CAD build for the part. Positions are in the model's coordinates, mm. Face numbers are marked on the shaded views. A direction names the side the tool comes from. Coordinates: 2 decimals unless noted, no trailing zeros. Loops run counter-clockwise (first coordinate to the right, second up) from the corner with the lowest first, then second, coordinate; pieces in that order, holes last. Notation, with made-up numbers: (8, 35) -> (43, 35) arc R14 ccw to (43, 52) -> close; hole circle Ø4 at (0.25, 72.25). An arc over 180 degrees is marked (long way). Return JSON: item names as keys, results as strings. Group by question number.
(1) Tool access for the marked faces 4 and 5: list every direction of +Z, -Z, +X, -X, +Y, -Y with a clear straight run to the whole face (end or side of a thin tool).
(2) Saw through at A-A on x = 10.5. Write the cut outline in (y, z).
(3) Saw through at D-D on y = -58. Write the cut outline in (x, z), then the cut area to 3 significant figures.
(4) Probe L1, parallel to X at y = -52.5, z = 52; L2, parallel to X at y = 41, z = 4; L3, parallel to Z at x = -36, y = -9.5. List the from-to ranges inside material, lowest first.
(5) Mould opens along Y. For the marked faces 1, 2 and 3 say: pulls with the +Y half, pulls with the -Y half, needs draft (parallel to the pull), parting line crosses it, or undercut.
(6) Flat gauge pins, fed straight in: pin 1 Ø4 at (x, y) = (0, -56) entering from -Z; pin 2 Ø5 at (x, y) = (41.5, 0) entering from +Z; pin 3 Ø6 at (x, y) = (2.5, 15.5) entering from +Z; pin 4 Ø6 at (x, y) = (-31, -28) entering from -Z. Where does each tip first touch, or does it go through?
(7) Saw through at B-B on y = 0. Give the number of separate pieces and of enclosed holes in the cut face, then the cut area to 3 significant figures.
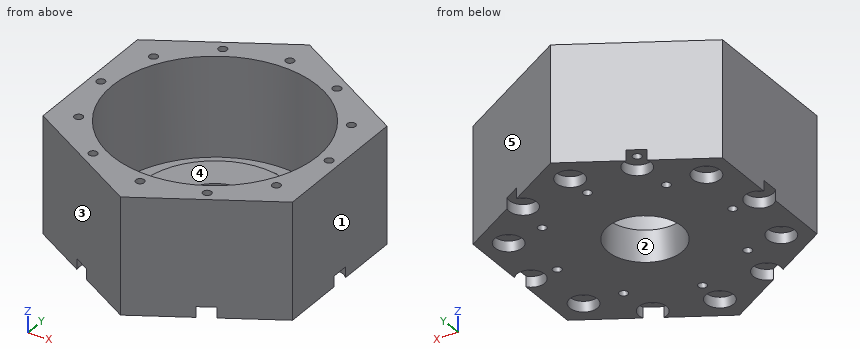
Autodesk Inventor part; units mm, degrees
ref_plane "YZ Plane" through (0, 0, 0) normal (1, 0, 0) x (0, 1, 0)
ref_plane "XZ Plane" through (0, 0, 0) normal (0, 1, 0) x (-1, 0, 0)
ref_plane "XY Plane" through (0, 0, 0) normal (0, 0, 1) x (1, 0, 0)
sketch "Sketch1" plane through (0, 0, 0) normal (0, 0, 1) x (1, 0, 0)
  circle A0 centre (0, 0) radius 17.5
  circle A1 centre (0, 0) radius 67.5
  circle A2 centre (41.5, 0) radius 2
  circle A3 centre (29.3449, 29.3449) radius 2
  circle A4 centre (0, 41.5) radius 2
  circle A5 centre (-29.3449, 29.3449) radius 2
  circle A6 centre (-41.5, 0) radius 2
  circle A7 centre (-29.3449, -29.3449) radius 2
  circle A8 centre (0, -41.5) radius 2
  circle A9 centre (29.3449, -29.3449) radius 2
  dimension "d0" = 35
  dimension "d1" = 135
  dimension "d2" = 4
  dimension "d3" = 41.5
  dimension "d6" = 360
extrude "Extrusion1" add sketch "Sketch1" along normal blind 15
sketch "Sketch5" plane through (0, 0, 15) normal (0, 0, 1) x (1, 0, 0)
  circle A0 centre (0, 0) radius 67.5
  circle A1 centre (0, 0) radius 48.5
  dimension "d19" = 97
extrude "Extrusion4" add sketch "Sketch5" along normal blind 40
sketch "Sketch8" plane through (0, 0, 55) normal (0, 0, 1) x (1, 0, 0)
  circle A0 centre (-54, 0) radius 2
  circle A1 centre (-46.7654, -27) radius 2
  circle A2 centre (-27, -46.7654) radius 2
  circle A3 centre (0, -54) radius 2
  circle A4 centre (27, -46.7654) radius 2
  circle A5 centre (46.7654, -27) radius 2
  circle A6 centre (54, 0) radius 2
  circle A7 centre (46.7654, 27) radius 2
  circle A8 centre (27, 46.7654) radius 2
  circle A9 centre (0, 54) radius 2
  circle A10 centre (-27, 46.7654) radius 2
  circle A11 centre (-46.7654, 27) radius 2
  point P0 (0, 0)
  dimension "d20" = 4
  dimension "d21" = 54
  dimension "d24" = 360
extrude "Extrusion5" cut sketch "Sketch8" against normal through all
sketch "Sketch11" plane through (0, 0, 55) normal (0, 0, 1) x (1, 0, 0)
  line L0 (0, 77.9423) -> (67.5, 38.9711)
  line L1 (67.5, 38.9711) -> (67.5, -38.9711)
  line L2 (67.5, -38.9711) -> (0, -77.9423)
  line L3 (0, -77.9423) -> (-67.5, -38.9711)
  line L4 (-67.5, -38.9711) -> (-67.5, 38.9711)
  line L5 (-67.5, 38.9711) -> (0, 77.9423)
  circle A0 centre (0, 0) radius 67.5
extrude "Extrusion8" add sketch "Sketch11" against normal blind 55 contours L0 A0 L5 | L0 L1 A0 | A0 L4 L5 | L1 L2 A0 | A0 L3 L4 | L2 L3 A0
sketch "Sketch12" plane through (0, 0, 0) normal (0, 0, -1) x (-1, 0, 0)
  circle A0 centre (-54, 0) radius 2
  circle A1 centre (-54, 0) radius 6.5
  circle A2 centre (-46.7654, -27) radius 6.5
  circle A3 centre (-27, -46.7654) radius 6.5
  circle A4 centre (0, -54) radius 6.5
  circle A5 centre (27, -46.7654) radius 6.5
  circle A6 centre (46.7654, -27) radius 6.5
  circle A7 centre (54, 0) radius 6.5
  circle A8 centre (46.7654, 27) radius 6.5
  circle A9 centre (27, 46.7654) radius 6.5
  circle A10 centre (0, 54) radius 6.5
  circle A11 centre (-27, 46.7654) radius 6.5
  circle A12 centre (-46.7654, 27) radius 6.5
  point P0 (0, 0)
  dimension "d37" = 13
  dimension "d40" = 360
extrude "Extrusion9" cut sketch "Sketch12" against normal blind 5 contours A0 | A1 | A2 | A3 | A4 | A5 | A6 | A7 | A8 | A9 | A10 | A11 | A12
sketch "Sketch16" plane through (0, 0, 15) normal (0, 0, 1) x (1, 0, 0)
  circle A0 centre (-41.5, 0) radius 2
  circle A1 centre (0, 0) radius 34.5
  circle A2 centre (0, 0) radius 48.5
  line L0 (-48.5, 0) -> (-34.5, 0)
  circle A3 centre (0, 0) radius 48.5
extrude "Extrusion11" cut sketch "Sketch16" against normal blind 7
sketch "Sketch19" plane through (0, 0, 55) normal (0, 0, 1) x (1, 0, 0)
  circle A0 centre (-27, 46.7654) radius 2
  circle A1 centre (27, 46.7654) radius 2
  circle A2 centre (54, 0) radius 2
  circle A3 centre (27, -46.7654) radius 2
  circle A4 centre (-27, -46.7654) radius 2
  circle A5 centre (-54, 0) radius 2
  circle A6 centre (-46.7654, -27) radius 2
  circle A7 centre (0, -54) radius 2
  circle A8 centre (46.7654, -27) radius 2
  circle A9 centre (46.7654, 27) radius 2
  circle A10 centre (0, 54) radius 2
  circle A11 centre (-46.7654, 27) radius 2
  circle A12 centre (0, 0) radius 48.5
  line L0 (0, -77.9423) -> (-67.5, -38.9711)
  line L1 (67.5, -38.9711) -> (0, -77.9423)
  line L2 (67.5, 38.9711) -> (67.5, -38.9711)
  line L3 (0, 77.9423) -> (67.5, 38.9711)
  line L4 (-67.5, 38.9711) -> (0, 77.9423)
  line L5 (-67.5, -38.9711) -> (-67.5, 38.9711)
  line L6 (0, 68.1273) -> (59, 34.0637)
  line L7 (59, 34.0637) -> (59, -34.0637)
  line L8 (59, -34.0637) -> (0, -68.1273)
  line L9 (0, -68.1273) -> (-59, -34.0637)
  line L10 (-59, -34.0637) -> (-59, 34.0637)
  line L11 (-59, 34.0637) -> (0, 68.1273)
  dimension "d58" = 118
extrude "Extrusion13" cut sketch "Sketch19" against normal through all contours L0 L5 L4 L3 L2 L1
properties part number "AC01" material "ABS Plastic"
Geometry results:
{
 "1": {"face 4": "+Z", "face 5": "+Z, -Z, +X, +Y"},
 "2": {"outline": "(-62.07, 0) -> (-14, 0) -> (-14, 15) -> (-32.86, 15) -> (-32.86, 8) -> (-47.35, 8) -> (-47.35, 55) -> (-62.07, 55) -> close; (14, 0) -> (62.07, 0) -> (62.07, 55) -> (47.35, 55) -> (47.35, 8) -> (32.86, 8) -> (32.86, 15) -> (14, 15) -> close"},
 "3": {"outline": "(-17.54, 0) -> (-5.12, 0) -> (-5.12, 5) -> (5.12, 5) -> (5.12, 0) -> (17.54, 0) -> (17.54, 55) -> (-17.54, 55) -> close", "area": "1,880 mm²"},
 "4": {"L1": "-27.07 to -1.32, 1.32 to 27.07", "L2": "-46.99 to -30, -24 to -1.94, 1.94 to 24, 30 to 46.99", "L3": "0 to 8"},
 "5": {"face 1": "needs draft", "face 2": "undercut", "face 3": "pulls with the -Y half"},
 "6": {"pin 1": "z = 5", "pin 2": "z = 8", "pin 3": "z = 15", "pin 4": "z = 0"},
 "7": {"separate pieces": "6", "enclosed holes": "0", "area": "1,310 mm²"}
}
